Geometry: see drawing. Coordinates: mm, zero at the bounding-box minimum. A direction names the side the tool comes from. Give positions to 0.01 mm unless a question says otherwise; leave off trailing zeros. Order: outer loops, then holes, each group sorted by start corner. A loop starts at its lowest first (then second) coordinate and runs counter-clockwise, first axis right, second up. Notation, with made-up numbers: (6, 77) -> (61, 77) arc R7 ccw to (61, 87) -> close; hole circle Ø9 at (45.25, -12.5). An arc over 180 degrees is marked (long way). Use one line per item in the form item = value. Start each with the question number.
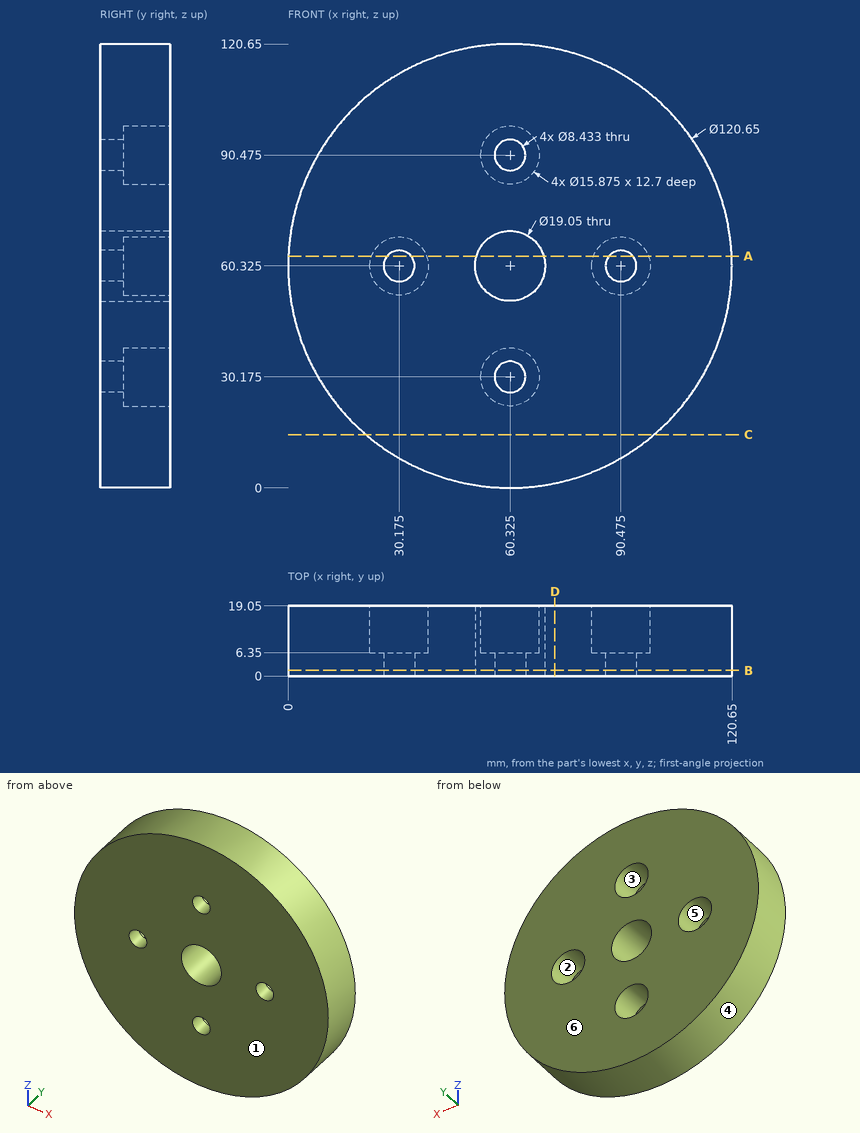
1) Draft query along X for the marked faces 1, 2, 3 and 4. Return one class per face: +X half, -X half, draft (parallel to the pull), parting line (faces both ways), or undercut.
2) Pin query (flat end, axial travel): pin 1 (13.5 mm diameter, centred on x = 90.47, z = 60.32, fed in from -Y); pin 2 (5 mm diameter, centred on x = 56, y = 5, fed in from +Z); pin 3 (1 mm diameter, centred on x = 33, y = 13, fed in from +Z); pin 4 (12.5 mm diameter, centred on x = 60.32, z = 90.47, fed in from +Y). Return the tip coordinate at first contact, or that it passes through.
3) Cut plane D-D, the plane x = 72.5. Return the cut outline in (y, z), plus the area to 3 significant figures.
4) Reachability of the marked faces 5 and 6 from +Z, -Z, +X, -X, +Y, -Y: full face, straight path, thin tool, end or side. Return the list, or none.
5) Cut plane C-C, the plane z = 14.5. Return the cut outline in (x, y).
6) Material intervals for probe 1 along Z at (x, y) = (61, 8.75); probe 2 along X at (y, z) = (7, 54.5); probe 3 along Z at (x, y) = (54, 15.25), sorted ascending.
7) Cut plane A-A, the plane z = 63. Return the cut outline in (x, y).
8) Cut plane B-B, the plane y = 1.5. Count the separate pieces of the cut face and the enclosed holes in it, plus the area to 3 significant figures.
Output values:
q1.face_1 = draft
q1.face_2 = undercut
q1.face_3 = undercut
q1.face_4 = parting line
q2.pin_1 = 0
q2.pin_2 = 120.62
q2.pin_3 = 114.36
q2.pin_4 = 6.35
q3.outline = (0, 1.24) -> (19.05, 1.24) -> (19.05, 119.41) -> (0, 119.41) -> close
q3.area = 2,250 mm^2
q4.face_5 = +Y
q4.face_6 = +Z, -Z, +X, -X, +Y
q5.outline = (21.09, 0) -> (99.56, 0) -> (99.56, 19.05) -> (21.09, 19.05) -> close
q6.probe_1 = 0 to 22.27, 38.08 to 50.82, 69.83 to 82.57, 98.38 to 120.65
q6.probe_2 = 0.28 to 24.78, 35.57 to 52.79, 67.86 to 85.08, 95.87 to 120.37
q6.probe_3 = 0.33 to 25.38, 34.97 to 53.2, 67.45 to 85.68, 95.27 to 120.32
q7.outline = (0.06, 0) -> (26.92, 0) -> (26.92, 6.35) -> (22.7, 6.35) -> (22.7, 19.05) -> (0.06, 19.05) -> close; (33.43, 0) -> (51.18, 0) -> (51.18, 19.05) -> (37.65, 19.05) -> (37.65, 6.35) -> (33.43, 6.35) -> close; (69.47, 0) -> (87.22, 0) -> (87.22, 6.35) -> (83, 6.35) -> (83, 19.05) -> (69.47, 19.05) -> close; (93.73, 0) -> (120.59, 0) -> (120.59, 19.05) -> (97.95, 19.05) -> (97.95, 6.35) -> (93.73, 6.35) -> close
q8.separate_pieces = 1
q8.enclosed_holes = 5
q8.area = 10,900 mm^2
